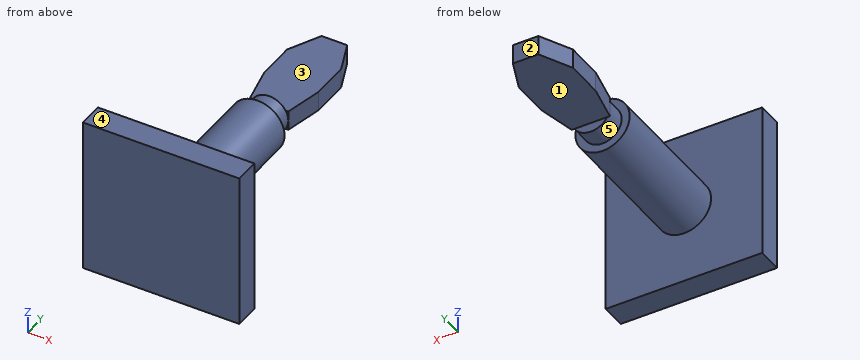
Autodesk Inventor part; units mm, degrees
ref_plane "YZ Plane" through (0, 0, 0) normal (1, 0, 0) x (0, 1, 0)
ref_plane "XZ Plane" through (0, 0, 0) normal (0, 1, 0) x (-1, 0, 0)
ref_plane "XY Plane" through (0, 0, 0) normal (0, 0, 1) x (1, 0, 0)
sketch "Sketch1" plane through (0, 0, 0) normal (0, 1, 0) x (-1, 0, 0)
  line L0 (6.35, 6.35) -> (-6.35, 6.35)
  line L1 (-6.35, 6.35) -> (-6.35, -6.35)
  line L2 (-6.35, -6.35) -> (6.35, -6.35)
  line L3 (6.35, -6.35) -> (6.35, 6.35)
  point P0 (0, 0)
  dimension "d0" = 12.7
  dimension "d1" = 12.7
  dimension "d2" = 6.35
  dimension "d3" = 6.35
extrude "Extrusion1" add sketch "Sketch1" along normal blind 2.032
sketch "Sketch2" plane through (0, 2.032, 0) normal (0, 1, 0) x (1, 0, 0)
  circle A0 centre (0, 0) radius 2.2
  dimension "d6" = 4.4
extrude "Extrusion2" add sketch "Sketch2" along normal blind 11.1
sketch "Sketch3" plane through (0, 13.132, 0) normal (0, 1, 0) x (1, 0, 0)
  circle A0 centre (0, 0) radius 1.55
  dimension "d9" = 3.1
extrude "Extrusion3" add sketch "Sketch3" along normal blind 1.6
sketch "Sketch4" plane through (0, 0, 0) normal (0, 0, 1) x (1, 0, 0)
  line L0 (-2.2, 23.432) -> (2.2, 23.432)
  line L1 (2.2, 23.432) -> (2.2, 14.732)
  line L2 (2.2, 14.732) -> (-2.2, 14.732)
  line L3 (-2.2, 14.732) -> (-2.2, 23.432)
  line L4 (-6.35, 0) -> (6.35, 0)
  line L5 (0, 0) -> (0, -2.1556)
  line L6 (1.55, 14.732) -> (2.2, 17.7603)
  line L7 (1.55, 14.732) -> (-1.55, 14.732)
  line L8 (-1.55, 14.732) -> (-2.2, 17.7603)
  line L9 (-0.9244, 23.432) -> (-2.2, 20.8496)
  line L10 (1.1495, 23.432) -> (2.2, 20.8496)
  dimension "d12" = 14.732
  dimension "d13" = 8.7
  dimension "d14" = 4.4
  dimension "d15" = 2.2
extrude "Extrusion4" add sketch "Sketch4" along normal mid plane 1.6 contours L0 L10 L1 L6 L2 L8 L3 L9
properties part number "11mm_Board_Support"
For this review, take the finished solid that the model builds, in its own axes (mm). Face numbers are marked on the shaded views. A direction names the side the tool comes from. Round coordinates to 2 decimals unless told otherwise and drop trailing zeros. Order: outer loops, then holes, each group sorted by start corner. A loop starts at its lowest first (then second) coordinate and runs counter-clockwise, first axis right, second up. Notation, with made-up numbers: (1, 35) -> (31, 35) arc R21 cw to (31, 72) -> close; hole circle Ø6 at (10, -5). An arc over 180 degrees is marked (long way). Write item = value, one per line. Start each with the question number.
1) Take a section at A-A on x = 0. State the section outline as (y, z) points, plus the area to 3 significant figures.
2) Take a section at D-D on y = 13.5. State the section outline as (x, z) points.
3) Take a section at C-C on y = 2.75. State the section outline as (x, z) points, plus the area to 3 significant figures.
4) To check wall thickness, follow line 1 (Y direction, x = -4.75, z = -0.75); line 2 (Z direction, x = 1.25, y = 15); line 3 (Y direction, x = -1, z = 1.5). State the ranges of each line that lie inside material, in increasing order. Write a range as from..to.
5) Insertion check: pin 1 (3.5 mm diameter, centred on x = 1, y = 19, fed in from +Z); pin 2 (4 mm diameter, centred on y = 6, z = 1, fed in from +X); pin 3 (6 mm diameter, centred on x = 5, y = 5.5, fed in from +Z). Each pin has a flat end and moves straight along its axis. Give the tip position at first contact, or say it passes through.
6) Tool access review of the marked faces 1, 2, 3, 4 and 5: name each direction out of +Z, -Z, +X, -X, +Y, -Y from which nothing blocks a thin tool from reaching the whole face with its end or side.
7) Take a section at B-B on z = 4. State the section outline as (x, y) points, plus the area to 3 significant figures.
Verdict:
q1.outline = (0, -6.35) -> (2.03, -6.35) -> (2.03, -2.2) -> (13.13, -2.2) -> (13.13, -1.55) -> (14.73, -1.55) -> (14.73, -0.8) -> (23.43, -0.8) -> (23.43, 0.8) -> (14.73, 0.8) -> (14.73, 1.55) -> (13.13, 1.55) -> (13.13, 2.2) -> (2.03, 2.2) -> (2.03, 6.35) -> (0, 6.35) -> close
q1.area = 93.5 mm2
q2.outline = circle Ø3.1 at (0, 0)
q3.outline = circle Ø4.4 at (0, 0)
q3.area = 15.2 mm2
q4.line_1 = 0..2.03
q4.line_2 = -0.8..0.8
q4.line_3 = 0..13.13
q5.pin_1 = 0.8
q5.pin_2 = 2.2
q5.pin_3 = 0.92
q6.face_1 = -Z, +X, -X, +Y
q6.face_2 = +Z, -Z, +X, -X, +Y
q6.face_3 = +Z, +X, -X, +Y
q6.face_4 = +Z, +X, -X, +Y, -Y
q6.face_5 = none
q7.outline = (-6.35, 0) -> (6.35, 0) -> (6.35, 2.03) -> (-6.35, 2.03) -> close
q7.area = 25.8 mm2
